Design review of the part built by this model. Coordinates are the model's own, in mm. A direction names the side the tool comes from. Coordinates: 2 decimals unless noted, no trailing zeros. Write each loop counter-clockwise with the first axis right and the second up, starting at its lowest first coordinate (ties: lowest second). Pieces come first, ordered by that corner, then holes.
Q1. Mouldability with a two-part tool opening along Z and no side actions: class faces 1 (the cylindrical face through (0.66, 35.493, 9.112)), 2 (the flat face through (0, -17, 1.5)), 3 (the cylindrical face through (29.4, -14.71, 18.43)) as pulls with the +Z half, pulls with the -Z half, needs draft (parallel to the pull), parting line crosses it, or undercut.
Q2. For probe 1 along Z at (x, y) = (-1, -27); probe 2 along X at (y, z) = (-23.5, 4); probe 3 along Y at (x, z) = (0, 20.7), list the stretches that pass through material, from the lowest coordinate up.
Q3. Insertion check: pin 1 (17 mm diameter, centred on x = 5, y = 11, fed in from -Z); pin 2 (6 mm diameter, centred on y = 17, z = 8, fed in from +X); pin 3 (8 mm diameter, centred on x = 16, z = 17.5, fed in from +Y); pin 4 (2 mm diameter, centred on x = -17, z = 14.5, fed in from -Y). Each pin has a flat end and moves straight along its axis. Give the tip position at first contact, or say it passes through.
Q4. Machinability: for faces 4 (the cylindrical face through (0.627, 33.993, 9.612)), 5 (the cylindrical face through (11.5, 27.7, 21)), 6 (the cylindrical face through (-4.769, -15.977, 0.761)), which of the approach directions +Z, -Z, +X, -X, +Y, -Y give a long, thin tool a straight path to every point of the face, cutting with its end or side? Answer none if there is none.
Q5. Take a section at B-B (z = 6.75). Give the boundary of the cut face in (x, y), and give its area (3 significant figures).
Q6. Take a section at A-A (x = 0). Give the boundary of the cut face in (y, z), and give its area (3 significant figures).
Q7. Take a section at C-C (x = -12). State how many separate pieces and enclosed holes the cut face has, and give its area (3 significant figures).
Autodesk Inventor part; units mm, degrees
ref_plane "РабПлоскость1" through (0, 5.5, 19) normal (0, -1, 0) x (0, 0, 1)
ref_plane "YZ Plane" through (0, 0, 0) normal (1, 0, 0) x (0, 1, 0)
ref_plane "XZ Plane" through (0, 0, 0) normal (0, 1, 0) x (-1, 0, 0)
sketch "Эскиз1" plane through (0, 0, 0) normal (0, 0, 1) x (1, 0, 0)
  line L0 (-30, -35.5) -> (30, -35.5)
  line L1 (30, -35.5) -> (30, 35.5)
  line L2 (30, 35.5) -> (-30, 35.5)
  line L3 (-30, 35.5) -> (-30, -35.5)
  line L4 (-30, -35.5) -> (30, 35.5) construction
  line L5 (30, -35.5) -> (-30, 35.5) construction
  point P0 (0, 0)
  dimension "d0" = 60
  dimension "d1" = 71
extrude "Выдавливание1" add sketch "Эскиз1" along normal blind 19
sketch "Эскиз2" plane through (0, 0, 19) normal (0, 0, 1) x (1, 0, 0)
  circle A0 centre (0, 5.5) radius 22 construction
  circle A1 centre (0, 5.5) radius 30
  line L0 (30, 35.5) -> (-30, 35.5)
  line L1 (-30, 35.5) -> (-30, -35.5)
  line L2 (30, -35.5) -> (30, 35.5)
  point P0 (0, 0)
  point P1 (30, 5.5)
  point P2 (0, 35.5)
  point P3 (-30, 5.5)
  dimension "d4" = 44
  dimension "d5" = 60
  dimension "d6" = 8
extrude "Выдавливание2" cut sketch "Эскиз2" against normal through all contours A1 L0 L2 | A1 L1 L0
sketch "Эскиз3" plane through (0, 0, 19) normal (0, 0, 1) x (1, 0, 0)
  circle A0 centre (0, 5.5) radius 25
  arc A1 (30, 5.5) -> (-30, 5.5) centre (0, 5.5) ccw
  circle A2 centre (0, 5.5) radius 22
  point P0 (0, 0)
  dimension "d9" = 50
  dimension "d10" = 44
extrude "Выдавливание3" add sketch "Эскиз3" along normal blind 4
fillet "Сопряжение1" radius 1.5 2 edges at (-25, 5.5, 19) (-25, 5.5, 23)
sketch "Эскиз4" plane through (0, 5.5, 19) normal (0, 0, 1) x (1, 0, 0)
  circle A0 centre (0, 0) radius 22
  point P0 (0, -5.5)
extrude "Выдавливание4" cut sketch "Эскиз4" against normal through all
sketch "Эскиз5" plane through (-30, -35.5, 0) normal (0, -1, 0) x (1, 0, 0)
  line L0 (1.5, 1.5) -> (58.5, 1.5)
  line L1 (58.5, 1.5) -> (58.5, 17.5)
  line L2 (58.5, 17.5) -> (1.5, 17.5)
  line L3 (1.5, 17.5) -> (1.5, 1.5)
  line L4 (60, 0) -> (60, 19)
  line L5 (0, 0) -> (60, 0)
  line L6 (0, 19) -> (60, 19)
  line L7 (0, 0) -> (0, 19)
  point P0 (30, 0)
  point P1 (30, 9.5)
  point P2 (30, 9.5)
  point P3 (60, 9.5)
  point P4 (30, 9.5)
  point P5 (30, 0)
  dimension "d16" = 1.5
  dimension "d17" = 1.5
  dimension "d18" = 1.5
  dimension "d19" = 1.5
ref_plane "РабПлоскость1" through (0, 5.5, 19) normal (0, -1, 0) x (0, 0, 1)
extrude "Выдавливание5" cut sketch "Эскиз5" against normal up to surface (41 mm away) contours L3 L2 L1 L0
sketch "Эскиз6" plane through (-28.5, 5.5, 17.5) normal (0, -1, 0) x (1, 0, 0)
  line L0 (6.5, 0) -> (6.5, -16)
  line L1 (0, 0) -> (6.5, 0)
  line L2 (0, -16) -> (0, 0)
  line L3 (6.5, -16) -> (0, -16)
  line L4 (28.5, -22.1) -> (28.5, 10.1)
  point P0 (28.5, -17.5)
revolve "Вращение1" cut sketch "Эскиз6" angle 180 about axis through (0, 5.5, 19) along (0, 0, -1)
fillet "Сопряжение2" radius 1 3 edges at (0, 35.5, 0) (30, -15, 0) (-30, -15, 0)
fillet "Сопряжение3" radius 2 3 edges at (0, 35.5, 19) (30, -15, 19) (-30, -15, 19)
equation "\"d17\" = d16"
equation "\"d18\" = d17"
equation "\"d19\" = d18"
properties part number "B6015L12F NF1" material "Стекло"
Response:
1. face 1: needs draft
1. face 2: undercut
1. face 3: pulls with the +Z half
2. probe 1: z = 0 to 1.5, 17.5 to 19
2. probe 2: x = -30 to -28.5, 28.5 to 30
2. probe 3: y = -19.5 to -16.5, 27.5 to 30.5
3. pin 1: passes through
3. pin 2: stops at x = 28.77
3. pin 3: stops at y = 32.98
3. pin 4: stops at y = 27.6
4. face 4: -Y
4. face 5: +Z
4. face 6: +Z, -Z
5. outline: (-30, -35.5) - (-28.5, -35.5) - (-28.5, 5.5) arc R28.5 cw to (28.5, 5.5) - (28.5, -35.5) - (30, -35.5) - (30, 5.5) arc R30 ccw to (-30, 5.5) - close
5. area: 261 mm2
6. outline: (-35.5, 0) - (-16.5, 0) - (-16.5, 1.5) - (-35.5, 1.5) - close; (-35.5, 17.5) - (-16.5, 17.5) - (-16.5, 23) - (-18, 23) arc R1.5 ccw to (-19.5, 21.5) - (-19.5, 20.5) arc R1.5 cw to (-21, 19) - (-35.5, 19) - close; (27.5, 0) - (34.5, 0) arc R1 ccw to (35.5, 1) - (35.5, 17) arc R2 ccw to (33.5, 19) - (32, 19) arc R1.5 cw to (30.5, 20.5) - (30.5, 21.5) arc R1.5 ccw to (29, 23) - (27.5, 23) - (27.5, 17.5) - (34, 17.5) - (34, 1.5) - (27.5, 1.5) - close
6. area: 128 mm2
7. separate pieces: 3
7. enclosed holes: 0
7. area: 148 mm2
